from build123d import *

# Parameters (mm, degrees)
SKETCH1_W                                       = 56.55
SKETCH1_H                                       = 197.425
BOSS_EXTRUDE1_DEPTH                             = 3.175
SKETCH2_R                                       = 5
CUT_EXTRUDE1_DEPTH                              = 103.731270343
SKETCH5_W                                       = 3.175
SKETCH5_H                                       = 197.425
BOSS_EXTRUDE2_DEPTH                             = 19.525
SKETCH14_W                                      = 76.075
SKETCH14_H                                      = 3.175
BOSS_EXTRUDE3_DEPTH                             = 3.175
M6_CLEARANCE_HOLE1_D                            = 6.6
CSK_FOR_M3_FLAT_HEAD_MACHINE_SCREW5_D           = 3.4
CSK_FOR_M3_FLAT_HEAD_MACHINE_SCREW5_CSINK_D     = 6.3
CSK_FOR_M3_FLAT_HEAD_MACHINE_SCREW5_CSINK_ANGLE = 90


with BuildPart() as part:
    # Sketch1 → Boss-Extrude1 (new body)
    with BuildSketch(Plane.XY):
        Rectangle(SKETCH1_W, SKETCH1_H)
    extrude(amount=BOSS_EXTRUDE1_DEPTH)

    # Sketch2 → Cut-Extrude1 (cut, through all)
    with BuildSketch(Plane(origin=(0, 0, 0), x_dir=(-1, 0, 0), z_dir=(0, 0, -1))):
        with Locations((-11.5, 30.630837161)):
            Circle(SKETCH2_R)
        with Locations((-11.5, 52.630837161)):
            Circle(SKETCH2_R)
        with Locations((-11.5, 41.630837161)):
            Circle(SKETCH2_R)
        with Locations((0, 52.630837161)):
            Circle(SKETCH2_R)
        with Locations((0, 41.630837161)):
            Circle(SKETCH2_R)
        with Locations((0, 30.630837161)):
            Circle(SKETCH2_R)
        with Locations((11.5, 30.630837161)):
            Circle(SKETCH2_R)
        with Locations((11.5, 41.630837161)):
            Circle(SKETCH2_R)
        with Locations((11.5, 52.630837161)):
            Circle(SKETCH2_R)
        with Locations((-11.5, -35.369162839)):
            Circle(SKETCH2_R)
        with Locations((-11.5, -13.369162839)):
            Circle(SKETCH2_R)
        with Locations((-11.5, -24.369162839)):
            Circle(SKETCH2_R)
        with Locations((0, -13.369162839)):
            Circle(SKETCH2_R)
        with Locations((0, -24.369162839)):
            Circle(SKETCH2_R)
        with Locations((0, -35.369162839)):
            Circle(SKETCH2_R)
        with Locations((11.5, -35.369162839)):
            Circle(SKETCH2_R)
        with Locations((11.5, -13.369162839)):
            Circle(SKETCH2_R)
        with Locations((11.5, -24.369162839)):
            Circle(SKETCH2_R)
    extrude(amount=-CUT_EXTRUDE1_DEPTH, mode=Mode.SUBTRACT)

    # Sketch5 → Boss-Extrude2 (add)
    with BuildSketch(Plane.ZY.offset(28.275)):
        with Locations((1.5875, 0)):
            Rectangle(SKETCH5_W, SKETCH5_H)
    extrude(amount=BOSS_EXTRUDE2_DEPTH)

    # Sketch14 → Boss-Extrude3 (add)
    with BuildSketch(Plane(origin=(0, 98.7125, 0), x_dir=(1, 0, 0), z_dir=(0, 1, 0))):
        with Locations((-9.7625, -1.5875)):
            Rectangle(SKETCH14_W, SKETCH14_H)
    extrude(amount=BOSS_EXTRUDE3_DEPTH)

    # M6 Clearance Hole1 (through all)
    with Locations(Plane.XY.offset(3.175)):
        with Locations((-17.4625, 92.3625001), (17.4625, 92.3625001), (17.4625, -78.8874999), (-17.4625, -78.8874999)):
            Hole(M6_CLEARANCE_HOLE1_D / 2)

    # CSK for M3 Flat Head Machine Screw5 (through all)
    with Locations(Plane(origin=(0, 0, 0), x_dir=(-1, 0, 0), z_dir=(0, 0, -1))):
        with Locations((0, -78.8874999), (0, 92.3625001)):
            CounterSinkHole(CSK_FOR_M3_FLAT_HEAD_MACHINE_SCREW5_D / 2, CSK_FOR_M3_FLAT_HEAD_MACHINE_SCREW5_CSINK_D / 2, counter_sink_angle=CSK_FOR_M3_FLAT_HEAD_MACHINE_SCREW5_CSINK_ANGLE)


solid = part.part
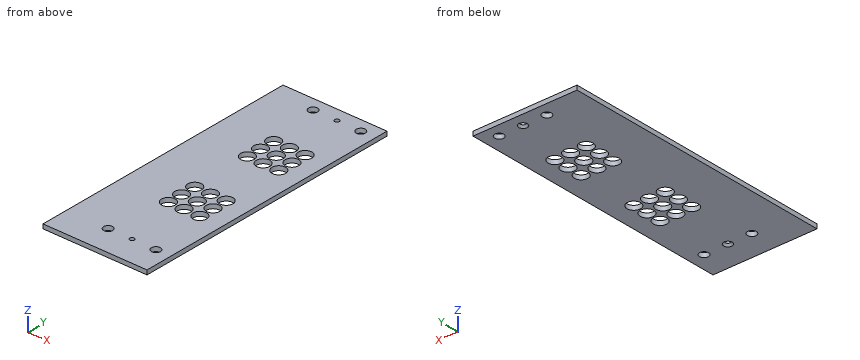
For this review, take the finished solid that the model builds, in its own axes (mm). Coordinates: 2 decimals unless noted, no trailing zeros. Order: outer loops, then holes, each group sorted by start corner. A loop starts at its lowest first (then second) coordinate and runs counter-clockwise, first axis right, second up. Notation, with made-up numbers: (-37, 66.25) - (10, 66.25) arc R27 ccw to (10, 86.25) - close; hole circle Ø5 at (-19.5, 76.5). An arc over 180 degrees is marked (long way). Answer as CSV lines item,"result". Start each with the question number.
1) Add section C-C (x = 9.5). State the section outline as (y, z) points (1 decimal).
2) Add section A-A (x = -11.5). State the section outline as (y, z) points (1 decimal).
3) Add section B-B (z = 2.65). Count the separate pieces of the cut face and the enclosed holes in it, then the cut area to 3 significant figures.
4) To check wall thickness, follow line 1 along Y through (x, z) = (-18.5, 1.6); line 2 along X through (y, z) = (-27.5, 1) (3 decimals); line 3 along Y through (x, z) = (-19, 2.45). State the ranges of each line that lie inside material, in increasing order. Write a range as [from, to].
Result:
1,outline,"(-98.7, 0) - (-40, 0) - (-40, 3.2) - (-98.7, 3.2) - close; (-30.8, 0) - (-29, 0) - (-29, 3.2) - (-30.8, 3.2) - close; (-19.8, 0) - (-18, 0) - (-18, 3.2) - (-19.8, 3.2) - close; (-8.8, 0) - (26, 0) - (26, 3.2) - (-8.8, 3.2) - close; (35.2, 0) - (37, 0) - (37, 3.2) - (35.2, 3.2) - close; (46.2, 0) - (48, 0) - (48, 3.2) - (46.2, 3.2) - close; (57.2, 0) - (101.9, 0) - (101.9, 3.2) - (57.2, 3.2) - close"
2,outline,"(-98.7, 0) - (-40.4, 0) - (-40.4, 3.2) - (-98.7, 3.2) - close; (-30.4, 0) - (-29.4, 0) - (-29.4, 3.2) - (-30.4, 3.2) - close; (-19.4, 0) - (-18.4, 0) - (-18.4, 3.2) - (-19.4, 3.2) - close; (-8.4, 0) - (25.6, 0) - (25.6, 3.2) - (-8.4, 3.2) - close; (35.6, 0) - (36.6, 0) - (36.6, 3.2) - (35.6, 3.2) - close; (46.6, 0) - (47.6, 0) - (47.6, 3.2) - (46.6, 3.2) - close; (57.6, 0) - (101.9, 0) - (101.9, 3.2) - (57.6, 3.2) - close"
3,separate pieces,"1"
3,enclosed holes,"24"
3,area,"13,700 mm^2"
4,line 1,"[-98.71, -82.02], [-75.75, 89.23], [95.5, 101.89]"
4,line 2,"[-47.8, -15.398], [-7.602, -3.898], [3.898, 7.602], [15.398, 28.275]"
4,line 3,"[-98.71, -81.81], [-75.97, 89.44], [95.28, 101.89]"
